The listing builds one solid part. Answer for the finished solid, in the listing's coordinates (mm). A direction names the side the tool comes from. Give positions to 0.01 mm unless a question says otherwise; leave off trailing zeros. Write each loop counter-clockwise with the first axis right and the second up, starting at its lowest first coordinate (ties: lowest second). Pieces come first, ordered by that corner, then holes. Notation, with made-up numbers: (-32, 4) - (-11, 4) arc R25 ccw to (-11, 17) - close; hole circle Ø5 at (-27, 85.25). An arc over 180 degrees is marked (long way). Return JSON: item names as keys, results as strings.
from build123d import *


with BuildPart() as f1:
    # F0 (on Front) → F1 (revolve)
    with BuildSketch(Plane.XZ):
        with BuildLine():
            Line((-18.796, 6.35), (0, 6.35))
            Line((0, 6.35), (0, 12.7))
            Line((0, 12.7), (-8.636, 12.7))
            ThreePointArc((-8.636, 12.7), (-10.252446, 13.369554), (-10.922, 14.986))
            Line((-10.922, 14.986), (-10.922, 17.399))
            ThreePointArc((-10.922, 17.399), (-14.195375, 25.301625), (-22.098, 28.575))
            Line((-22.098, 28.575), (-91.186, 28.575))
            ThreePointArc((-91.186, 28.575), (-92.802446, 29.244554), (-93.472, 30.861))
            Line((-93.472, 30.861), (-93.472, 35.814))
            ThreePointArc((-93.472, 35.814), (-94.141554, 37.430446), (-95.758, 38.1))
            Line((-95.758, 38.1), (-103.124, 38.1))
            Line((-103.124, 38.1), (-103.124, 34.925))
            Line((-103.124, 34.925), (-100.838, 34.925))
            Line((-100.838, 34.925), (-100.838, 22.225))
            Line((-100.838, 22.225), (-71.374, 22.225))
            Line((-71.374, 22.225), (-71.374, 6.35))
            Line((-71.374, 6.35), (-65.024, 6.35))
            Line((-65.024, 6.35), (-65.024, 22.225))
            Line((-65.024, 22.225), (-18.796, 22.225))
            Line((-18.796, 22.225), (-18.796, 6.35))
        make_face()
    revolve(axis=Axis((-51.562, 0, 0), (1, 0, 0)))


solid = f1.part
Item 1: A cutting plane is placed at B-B on x = -16. Determine the outline of the cut face in (y, z), then the cut area to 3 significant figures.
Answer below:
{"outline": "circle Ø53.53 at (0, 0); hole circle Ø12.7 at (0, 0)", "area": "2,120 mm²"}
Item 2: A cutting plane is placed at A-A on x = -77.5. Determine the outline of the cut face in (y, z) (3 decimals).
Answer below:
{"outline": "circle Ø57.15 at (0, 0); hole circle Ø44.45 at (0, 0)"}
Item 3: For faces 4 (the face through (-65.024, 5, -5)), 5 (the face through (-101.965, 21.251, -27.715)), 6 (the face through (-4.38, 12.4, -2.75)), determine the directions among +Z, -Z, +X, -X, +Y, -Y from which every point of the face is accessible in a straight line to the end or side of a thin tool.
Answer below:
{"face 4": "none", "face 5": "-X", "face 6": "+X"}
Item 4: The mould has two halves that part along X. Classify faces 1 (the face through (-18.796, 5, 5)), 2 (the face through (-9.27, 6.2, -1.38)), 3 (the face through (-100.838, 23, 0)): +X half, -X half, draft (parallel to the pull), parting line (faces both ways), or undercut.
Answer below:
{"face 1": "undercut", "face 2": "draft", "face 3": "-X half"}
Item 5: Consider L1, parallel to Z at x = -7.5, y = 0; L2, parallel to Y at x = -35, z = 0 (3 decimals); L3, parallel to Z at x = -70, y = 0 (3 decimals). Determine where each line is inside the solid, lowest interval first.
Answer below:
{"L1": "z = -12.7 to -6.35, 6.35 to 12.7", "L2": "y = -28.575 to -22.225, 22.225 to 28.575", "L3": "z = -28.575 to -6.35, 6.35 to 28.575"}
Item 6: Flat-ended cylindrical pins translate along their axes: P1, Ø4, axis at x = -27.5, z = -16.5, coming from the -Y side; P2, Ø8, axis at x = -24, z = 20, coming from the +Y side; P3, Ø13.5, axis at y = 6, z = 2, coming from the -X side. Find the tip coordinate at first contact, or state that the pin passes through.
Answer below:
{"P1": "stops at y = -24.62", "P2": "stops at y = 23.68", "P3": "stops at x = -71.37"}
